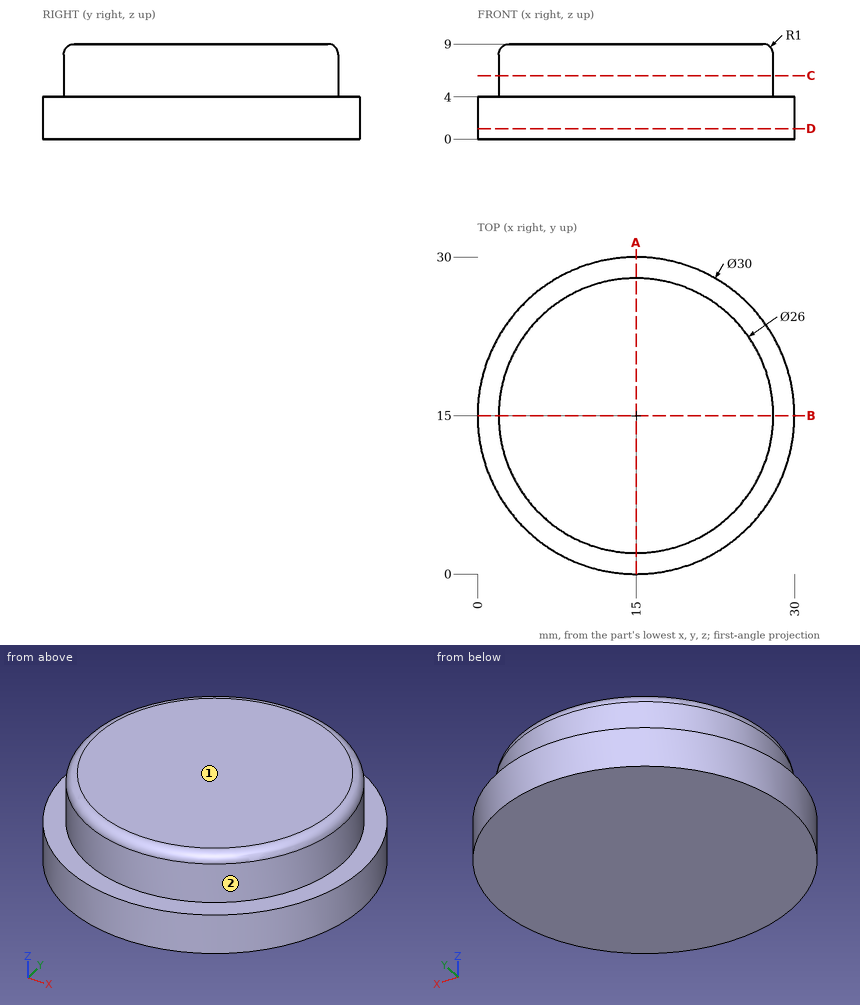
Source: three-view drawing plus pictorial views. Frame: mm from the lowest corner of the part. A direction names the side the tool comes from. Coordinates: 2 decimals unless noted, no trailing zeros. Order: outer loops, then holes, each group sorted by start corner. A loop starts at its lowest first (then second) coordinate and runs counter-clockwise, first axis right, second up. Notation, with made-up numbers: M 53,9 L 74,9 A24 cw 74,44 Z; hole C 75.5,18 d11. An arc over 180 degrees is marked long. Write each question's results on one line, items separated by ' | '. Start each with the question number.
1. Section A-A, the plane x = 15. Return the cut outline in (y, z).
2. Material intervals for L1, parallel to Z at x = 25.5, y = 7.25; L2, parallel to X at y = 10, z = 4.75; L3, parallel to Y at x = 19, z = 7, sorted ascending.
3. Reachability of the marked faces 1 and 2 from +Z, -Z, +X, -X, +Y, -Y: full face, straight path, thin tool, end or side. Return the list, or none.
4. Section C-C, the plane z = 6. Return the cut outline in (x, y), then the cut area to 3 significant figures.
5. Pin query (flat end, axial travel): pin 1 (3 mm diameter, centred on y = 7.5, z = 3, fed in from +X); pin 2 (1.5 mm diameter, centred on x = 6, z = 7, fed in from -Y); pin 3 (2 mm diameter, centred on x = 8.5, z = 6, fed in from -Y). Return the tip coordinate at first contact, or that it passes through.
6. Section D-D, the plane z = 1. Return the cut outline in (x, y), then the cut area to 3 significant figures.
Solution:
1) outline: M 0,0 L 30,0 L 30,4 L 28,4 L 28,8 A1 ccw 27,9 L 3,9 A1 ccw 2,8 L 2,4 L 0,4 Z
2) L1: 0 to 4 | L2: 3 to 27 | L3: 2.63 to 27.37
3) face 1: +Z, +X, -X, +Y, -Y | face 2: +Z
4) outline: C 15,15 d26 | area: 531 mm²
5) pin 1: x = 28.75 | pin 2: y = 4.95 | pin 3: y = 3.22
6) outline: C 15,15 d30 | area: 707 mm²
